Check sheet for the drawn part. Datum: minimum x, y, z corner. Units: mm. Give positions to 0.01 mm unless a question says otherwise; leave off trailing zeros. Order: outer loops, then holes, each group sorted by start corner. A loop starts at its lowest first (then second) coordinate and runs counter-clockwise, first axis right, second up. Notation, with made-up numbers: M -32,21.5 L -2,21.5 A16 ccw -2,47.5 Z; hole C 38.5,73 d3. An arc over 180 degrees is marked long. Answer as CSV lines item,"result". Start each with the question number.
Q1. Section check D-D, the plane z = 40. Record the boundary of the cut face in (x, y).
Q2. Thickness scan on line 1 (Y direction, x = 1.7, z = 55); line 2 (Y direction, x = 2.9, z = 52). Record the ranges inside material, lowest first.
Q3. Go/stop test with flat-tipped pins: pin 1 (2 mm diameter, centred on x = 2, y = 3.5, fed in from -Z); pin 2 (1.2 mm diameter, centred on x = 2, z = 16.5, fed in from -Y); pin 3 (1.2 mm diameter, centred on x = 2, y = 1.5, fed in from +Z). Record where each tip stops, or that it passes through.
Q4. Section check A-A, the plane z = 55. Record the boundary of the cut face in (x, y).
Q5. Section check C-C, the plane x = 2.1. Record the boundary of the cut face in (y, z), then the cut area to 3 significant figures.
Q6. Section check B-B, the plane y = 8. Record the boundary of the cut face in (x, z), then the cut area to 3 significant figures.
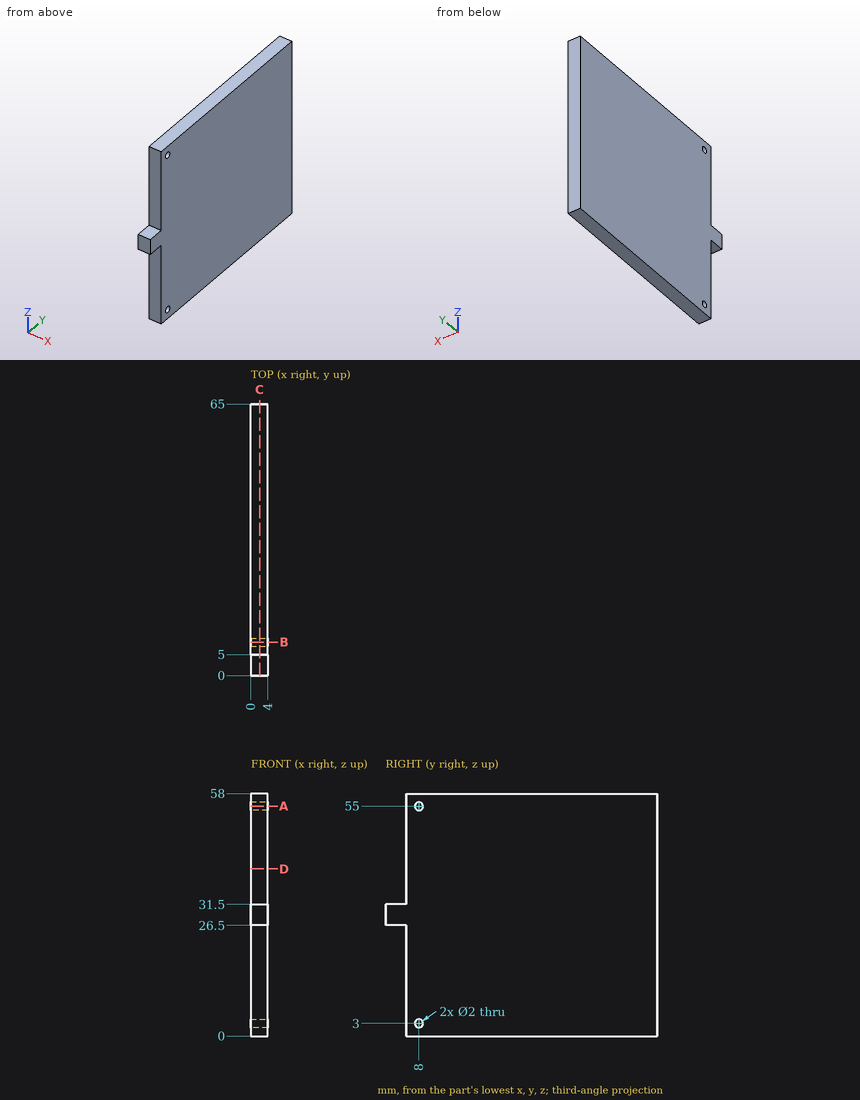
Answer block:
1,outline,"M 0,5 L 4,5 L 4,65 L 0,65 Z"
2,line 1,"y = 5 to 7, 9 to 65"
2,line 2,"y = 5 to 65"
3,pin 1,"stops at z = 26.5"
3,pin 2,"stops at y = 5"
3,pin 3,"stops at z = 31.5"
4,outline,"M 0,5 L 4,5 L 4,7 L 0,7 Z; M 0,9 L 4,9 L 4,65 L 0,65 Z"
5,outline,"M 0,26.5 L 5,26.5 L 5,0 L 65,0 L 65,58 L 5,58 L 5,31.5 L 0,31.5 Z; hole C 8,3 d2; hole C 8,55 d2"
5,area,"3,500 mm2"
6,outline,"M 0,0 L 4,0 L 4,2 L 0,2 Z; M 0,4 L 4,4 L 4,54 L 0,54 Z; M 0,56 L 4,56 L 4,58 L 0,58 Z"
6,area,"216 mm2"
